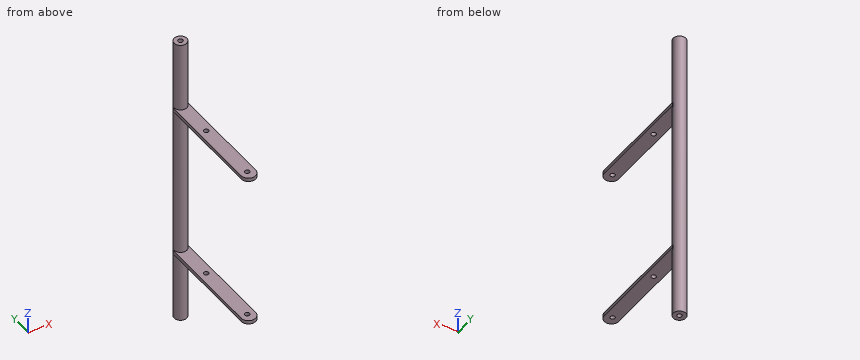
from build123d import *

# Parameters (mm, degrees)
SKETCH1_R           = 17.5
BOSS_EXTRUDE1_DEPTH = 415
CUT_EXTRUDE1_REACH  = 832.369
SKETCH2_R           = 6.5
SKETCH3_W           = 10
SKETCH3_H           = 317.5
BOSS_EXTRUDE2_DEPTH = 20
FILLET1_R           = 20
SKETCH4_R           = 6.5
CUT_EXTRUDE2_DEPTH  = 542


with BuildPart() as part:
    # Sketch1 → Boss-Extrude1 (new, symmetric)
    with BuildSketch(Plane.XY):
        Circle(SKETCH1_R)
    extrude(amount=BOSS_EXTRUDE1_DEPTH, both=True)

    # Sketch2 → Cut-Extrude1 (cut, up to next)
    with BuildSketch(Plane.XY.offset(415), mode=Mode.PRIVATE) as cut_extrude1_sk1:
        Circle(SKETCH2_R)
    cut_extrude1_tool1 = extrude(cut_extrude1_sk1.sketch, amount=-CUT_EXTRUDE1_REACH, mode=Mode.PRIVATE) & part.part
    add(cut_extrude1_tool1.solids().sort_by_distance((0, 0, 415))[0], mode=Mode.SUBTRACT)

    # Sketch3 → Boss-Extrude2 (add, symmetric)
    with BuildSketch(Plane(origin=(0, 0, 0), x_dir=(0, 0, -1), z_dir=(1, 0, 0))):
        with Locations((-215, -158.75)):
            Rectangle(SKETCH3_W, SKETCH3_H)
        with Locations((215, -158.75)):
            Rectangle(SKETCH3_W, SKETCH3_H)
    extrude(amount=BOSS_EXTRUDE2_DEPTH, both=True)

    # Fillet1
    fillet1_edges = [part.edges().sort_by_distance(p)[0] for p in [
        (-20, -317.5, -215),
        (20, -317.5, -215),
        (-20, -317.5, 215),
        (20, -317.5, 215),
    ]]
    fillet(fillet1_edges, radius=FILLET1_R - 0.0001)  # a hair under: the kernel refuses the full size

    # Sketch4 → Cut-Extrude2 (cut)
    with BuildSketch(Plane.XY.offset(220)):
        with Locations(Location((0, -292.5, 0), (0, 0, 270))):
            Circle(SKETCH4_R)
        with Locations(Location((0, -112.5, 0), (0, 0, 270))):
            Circle(SKETCH4_R)
    extrude(amount=-CUT_EXTRUDE2_DEPTH, mode=Mode.SUBTRACT)


solid = part.part
The model under review builds one solid part; all positions refer to its coordinate system, in mm. Round coordinates to 2 decimals unless told otherwise and drop trailing zeros. Loops run counter-clockwise (first coordinate to the right, second up) from the corner with the lowest first, then second, coordinate; pieces in that order, holes last. Notation, with made-up numbers: M -2.75,50 L 38.25,50 A4 cw 38.25,56 Z; hole C 28.5,-27 d3. An arc over 180 degrees is marked long. Answer as CSV lines item,"result". Start each with the question number.
Item 1: Wall thickness on line 1 (Z direction, x = -7.5, y = -148); line 2 (Y direction, x = 0, z = -81); line 3 (X direction, y = -112, z = -214): over which ranges is each line inside the solid? List them lowest first. Write a range as [from, to].
Item 2: Consider section B-B (z = -17). Write out the cut boundary in (x, y), then the cut area to 3 significant figures.
Item 3: Insertion check: P1, Ø1, axis at x = 5, y = -201.5, coming from the -Z side; P2, Ø20, axis at x = 8.5, y = -85.5, coming from the +Z side; P3, Ø0.8, axis at x = 19, z = 215, coming from the +Y side. Each pin has a flat end and moves straight along its axis. Give the tip position at first contact, or say it passes through.
Item 4: Consider section A-A (y = -68.5). Write out the cut boundary in (x, z), then the cut area to 3 significant figures.
Answer:
1,line 1,"z = [-220, -210], [210, 220]"
1,line 2,"y = [-17.5, -6.5], [6.5, 17.5]"
1,line 3,"x = [-20, -6.48], [6.48, 20]"
2,outline,"C 0,0 d35; hole C 0,0 d13"
2,area,"829 mm^2"
3,P1,"stops at z = -220"
3,P2,"stops at z = 220"
3,P3,"stops at y = 0"
4,outline,"M -20,-220 L 20,-220 L 20,-210 L -20,-210 Z; M -20,210 L 20,210 L 20,220 L -20,220 Z"
4,area,"800 mm^2"
